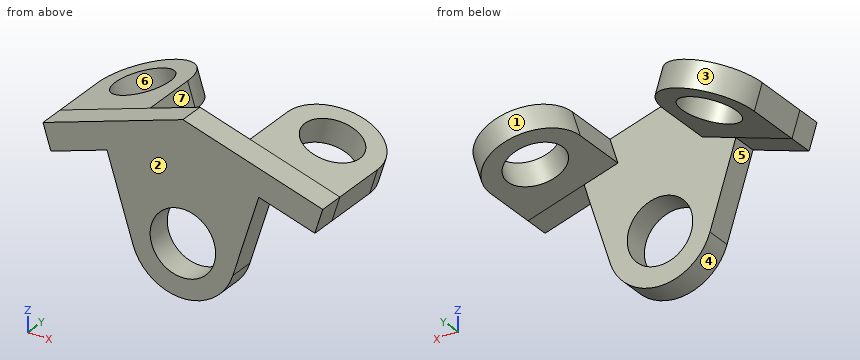
```python
from build123d import *

# Parameters (mm, degrees)
SKETCH1_R           = 12.5
BOSS_EXTRUDE1_DEPTH = 10
SKETCH2_R           = 11
BOSS_EXTRUDE2_DEPTH = 10
SKETCH4_R           = 11
BOSS_EXTRUDE3_DEPTH = 10


with BuildPart() as part:
    # Sketch1 → Boss-Extrude1 (new body)
    with BuildSketch(Plane(origin=(0, 0, 0), x_dir=(1, 0, 0), z_dir=(0, 1, 0))):
        with BuildLine():
            Line((0, 0), (53.408149242, 16.839524772))
            Line((53.408149242, 16.839524772), (50.401091247, 26.37669428))
            Line((50.401091247, 26.37669428), (28.972750838, 19.620364501))
            Line((28.972750838, 19.620364501), (19.074339015, 51.01411599))
            ThreePointArc((19.074339015, 51.01411599), (0, 65), (-19.074339015, 51.01411599))
            Line((-19.074339015, 51.01411599), (-28.972750838, 19.620364501))
            Line((-28.972750838, 19.620364501), (-50.401091247, 26.37669428))
            Line((-50.401091247, 26.37669428), (-53.408149242, 16.839524772))
            Line((-53.408149242, 16.839524772), (0, 0))
        make_face()
        with Locations((0, 45)):
            Circle(SKETCH1_R, mode=Mode.SUBTRACT)
    extrude(amount=BOSS_EXTRUDE1_DEPTH)

    # Sketch2 → Boss-Extrude2 (add)
    with BuildSketch(Plane(origin=(0, 0, 0), x_dir=(0.953716951, 0, -0.3007058), z_dir=(0.3007058, 0, 0.953716951))):
        with BuildLine():
            Line((56, 32), (56, 10))
            Line((56, 10), (20, 10))
            Line((20, 10), (20, 32))
            ThreePointArc((20, 32), (38, 50), (56, 32))
        make_face()
        with Locations((38, 32)):
            Circle(SKETCH2_R, mode=Mode.SUBTRACT)
    extrude(amount=-BOSS_EXTRUDE2_DEPTH)

    # Sketch4 → Boss-Extrude3 (add)
    with BuildSketch(Plane(origin=(0, 0, 0), x_dir=(0.953716951, 0, 0.3007058), z_dir=(-0.3007058, 0, 0.953716951))):
        with BuildLine():
            Line((-20, 10), (-20, 32))
            ThreePointArc((-20, 32), (-38, 50), (-56, 32))
            Line((-56, 32), (-56, 10))
            Line((-56, 10), (-20, 10))
        make_face()
        with Locations((-38, 32)):
            Circle(SKETCH4_R, mode=Mode.SUBTRACT)
    extrude(amount=-BOSS_EXTRUDE3_DEPTH)


solid = part.part
```
Geometry check sheet. Reference: the model listing, model coordinates, mm. Face numbers are marked on the shaded views. A direction names the side the tool comes from. Round coordinates to 2 decimals unless told otherwise and drop trailing zeros. Order: outer loops, then holes, each group sorted by start corner. A loop starts at its lowest first (then second) coordinate and runs counter-clockwise, first axis right, second up. Notation, with made-up numbers: (-13, 74.25) - (37, 74.25) arc R19 ccw to (37, 105.25) - close; hole circle Ø1 at (85, 80.25). An arc over 180 degrees is marked (long way). Use a Markdown table: item, result. Add a question column.
(1) Material ranges on line 1 along Z through (x, y) = (0, 5.5); line 2 along Y through (x, z) = (11, -10); line 3 along X through (y, z) = (7, -45), recorded low to high. Write a range as [from, to].
(2) Release check for a two-part mould opening along X. For the marked faces 1, 2, 3 and 4 record: pulls with the +X half, pulls with the -X half, needs draft (parallel to the pull), parting line crosses it, or undercut.
(3) Sectioned sample at D-D, the plane y = 39. Enter the section's corners in (x, z), and give its area (3 significant figures).
(4) Depth check by flat-ended pin: pin 1 (3 mm diameter, centred on x = -30.5, z = -11, fed in from +Y); pin 2 (2 mm diameter, centred on x = -37, y = 13.5, fed in from +Z); pin 3 (2 mm diameter, centred on x = -27.5, z = -9, fed in from +Y). Enter the tip coordinate at first touch or a pass-through.
(5) Sectioned sample at B-B, the plane y = 3.5. Enter the section's corners in (x, z), and give its area (3 significant figures).
(6) Sectioned sample at C-C, the plane z = -55. Enter the section's corners in (x, y), and give its area (3 significant figures).
(7) Tool access check on the marked faces 5, 6 and 7. Record the directions out of +Z, -Z, +X, -X, +Y, -Y that give a thin tool (end or side, any length) a straight path to the whole face; none if there is none.
(8) Sectioned sample at A-A, the plane y = 14.5. Enter the section's corners in (x, z).
Answers below:
| question | item | result |
|---|---|---|
| 1 | line 1 | [-65, -57.5], [-32.5, 0] |
| 1 | line 2 | [0, 10] |
| 1 | line 3 | [-20.97, -12.5], [12.5, 20.97] |
| 2 | face 1 | undercut |
| 2 | face 2 | needs draft |
| 2 | face 3 | undercut |
| 2 | face 4 | parting line crosses it |
| 3 | outline | (-52.06, -16.41) - (-49.05, -25.95) - (-41.33, -23.52) - (-44.33, -13.98) - close; (-28.15, -8.88) - (-25.14, -18.41) - (-17.42, -15.98) - (-20.43, -6.44) - close; (17.42, -15.98) - (25.14, -18.41) - (28.15, -8.88) - (20.43, -6.44) - close; (41.33, -23.52) - (49.05, -25.95) - (52.06, -16.41) - (44.33, -13.98) - close |
| 3 | area | 324 mm² |
| 4 | pin 1 | y = 49.53 |
| 4 | pin 2 | z = -11.35 |
| 4 | pin 3 | y = 48.09 |
| 5 | outline | (-53.41, -16.84) - (-50.4, -26.38) - (-28.97, -19.62) - (-19.07, -51.01) arc R20 ccw to (19.07, -51.01) - (28.97, -19.62) - (50.4, -26.38) - (53.41, -16.84) - (0, 0) - close; hole circle Ø25 at (0, -45) |
| 5 | area | 2,760 mm² |
| 6 | outline | (-17.32, 0) - (-7.5, 0) - (-7.5, 10) - (-17.32, 10) - close; (7.5, 0) - (17.32, 0) - (17.32, 10) - (7.5, 10) - close |
| 6 | area | 196 mm² |
| 7 | face 5 | -Z, +Y, -Y |
| 7 | face 6 | none |
| 7 | face 7 | +Z, +Y |
| 8 | outline | (-53.41, -16.84) - (-50.4, -26.38) - (-16.07, -15.55) - (-19.07, -6.01) - close; (16.07, -15.55) - (50.4, -26.38) - (53.41, -16.84) - (19.07, -6.01) - close |
